Work out the finished part from the listing and answer in its coordinate system (mm). Face numbers are marked on the shaded views. A direction names the side the tool comes from. Give positions to 0.01 mm unless a question says otherwise; leave off trailing zeros. Loops run counter-clockwise (first coordinate to the right, second up) from the corner with the lowest first, then second, coordinate; pieces in that order, holes last. Notation, with made-up numbers: M -21,78.25 L 3,78.25 A14 cw 3,86.25 Z; hole C 53.25,20 d10. An arc over 180 degrees is marked long. Write item = value, one per line. Start each with the question number.
1. For the marked faces 4, 5, 6 and 7, determine the directions among +Z, -Z, +X, -X, +Y, -Y from which every point of the face is accessible in a straight line to the end or side of a thin tool.
2. Section D-D on x = 4.75 is taken. Determine the outline of the cut face in (y, z), plus the area to 3 significant figures.
3. Section A-A on x = 0 is taken. Determine the outline of the cut face in (y, z) (3 decimals), plus the area to 3 significant figures.
4. Flat-ended cylindrical pins translate along their axes: pin 1 Ø1.6 at (x, z) = (-5.5, 8.5) entering from +Y; pin 2 Ø1.5 at (x, y) = (4.5, 1.5) entering from +Z; pin 3 Ø0.8 at (y, z) = (4, -5) entering from -X. Find the tip coordinate at first contact, or state that the pin passes through.
5. Consider L1, parallel to Z at x = 4.75, y = 3.3; L2, parallel to Z at x = 2.25, y = 4.2; L3, parallel to X at y = 1.15, z = 0 (3 decimals). Determine where each line is inside the solid, lowest interval first. Write a range as [from, to].
6. Section C-C on z = 10.5 is taken. Determine the outline of the cut face in (x, y).
7. The mould has two halves that part along Z. Classify the marked faces 1, 2 and 3: released by +Z, released by -Z, zero draft, split by the parting line, or undercut.
8. Section B-B on z = 3.5 is taken. Determine the outline of the cut face in (x, y).
```python
from build123d import *

# Parameters (mm, degrees)
CROQUIS1_W              = 20
CROQUIS1_H              = 20
SALIENTE_EXTRUIR1_DEPTH = 3
CROQUIS2_W              = 14
CROQUIS2_H              = 14
SALIENTE_EXTRUIR2_DEPTH = 2
CROQUIS3_W              = 12
CROQUIS3_H              = 12
CORTAR_EXTRUIR1_DEPTH   = 2
CROQUIS4_W              = 6
CROQUIS4_H              = 2.600399467
CORTAR_EXTRUIR2_DEPTH   = 3
SALIENTE_EXTRUIR3_DEPTH = 3
CROQUIS6_W              = 3
CROQUIS6_H              = 3
CROQUIS6_W_2            = 2
CROQUIS6_H_2            = 2
CROQUIS6_W_3            = 4
SALIENTE_EXTRUIR4_DEPTH = 0.5
CROQUIS7_W              = 6
CROQUIS7_H              = 2.831475003
CORTAR_EXTRUIR3_DEPTH   = 1
CROQUIS8_W              = 1
CROQUIS8_H              = 5.440516932
SALIENTE_EXTRUIR5_DEPTH = 0.5
CROQUIS10_W             = 3
CROQUIS10_H             = 4.43187447
CROQUIS10_W_2           = 2
CROQUIS10_H_2           = 3.43187447
CROQUIS10_H_3           = 3.13625106
CROQUIS10_H_4           = 2.13625106
CROQUIS10_H_5           = 2.43247793
CROQUIS10_H_6           = 1.43247793
CROQUIS10_W_3           = 1.053408661
CROQUIS10_W_4           = 3.858734252
CROQUIS10_W_5           = 5
CROQUIS10_W_6           = 2.087857087
CROQUIS10_W_7           = 1.087857087
CROQUIS10_H_7           = 1.99939654
CROQUIS10_H_8           = 0.99939654
SALIENTE_EXTRUIR6_DEPTH = 1.5
CROQUIS11_W             = 6
CROQUIS11_H             = 5.43187447
SALIENTE_EXTRUIR7_DEPTH = 1.5
CROQUIS12_R             = 1.575
CORTAR_EXTRUIR4_DEPTH   = 2.5


with BuildPart() as part:
    # Croquis1 → Saliente-Extruir1 (new body)
    with BuildSketch(Plane(origin=(0, 0, 0), x_dir=(1, 0, 0), z_dir=(0, 1, 0))):
        Rectangle(CROQUIS1_W, CROQUIS1_H)
    extrude(amount=SALIENTE_EXTRUIR1_DEPTH)

    # Croquis2 → Saliente-Extruir2 (add)
    with BuildSketch(Plane(origin=(0, 3, 0), x_dir=(1, 0, 0), z_dir=(0, 1, 0))):
        Rectangle(CROQUIS2_W, CROQUIS2_H)
    extrude(amount=SALIENTE_EXTRUIR2_DEPTH)

    # Croquis3 → Cortar-Extruir1 (cut)
    with BuildSketch(Plane(origin=(0, 5, 0), x_dir=(1, 0, 0), z_dir=(0, 1, 0))):
        Rectangle(CROQUIS3_W, CROQUIS3_H)
    extrude(amount=-CORTAR_EXTRUIR1_DEPTH, mode=Mode.SUBTRACT)

    # Croquis4 → Cortar-Extruir2 (cut)
    with BuildSketch(Plane(origin=(0, 5, 0), x_dir=(1, 0, 0), z_dir=(0, 1, 0))):
        with Locations((0, -5.699800267)):
            Rectangle(CROQUIS4_W, CROQUIS4_H)
    extrude(amount=-CORTAR_EXTRUIR2_DEPTH, mode=Mode.SUBTRACT)

    # Croquis5 → Saliente-Extruir3 (add)
    with BuildSketch(Plane(origin=(0, 0, 0), x_dir=(1, 0, 0), z_dir=(0, 1, 0))):
        Polygon((-3, -10), (-1.049339158, -10), (-1.049339158, -14.469917755), (-2.287906915, -14.469917755), align=None)
        Polygon((0.678136925, -10), (3, -10), (1.818923018, -14.469917755), (0.678136925, -14.469917755), align=None)
    extrude(amount=SALIENTE_EXTRUIR3_DEPTH)

    # Croquis6 → Saliente-Extruir4 (add)
    # profile 1 of 4: a face of its own
    with BuildSketch(Plane(origin=(0, 3, 0), x_dir=(1, 0, 0), z_dir=(0, 1, 0))):
        with Locations((-8.5, -8.5)):
            Rectangle(CROQUIS6_W, CROQUIS6_H)
        with Locations((-8.5, -8.5)):
            Rectangle(CROQUIS6_W_2, CROQUIS6_H_2, mode=Mode.SUBTRACT)
    # profile 2 of 4: a face of its own
    with BuildSketch(Plane(origin=(0, 3, 0), x_dir=(1, 0, 0), z_dir=(0, 1, 0))):
        with Locations((-5, -8.5)):
            Rectangle(CROQUIS6_W_3, CROQUIS6_H)
        with Locations((-5, -8.5)):
            Rectangle(CROQUIS6_W, CROQUIS6_H_2, mode=Mode.SUBTRACT)
    # profile 3 of 4: a face of its own
    with BuildSketch(Plane(origin=(0, 3, 0), x_dir=(1, 0, 0), z_dir=(0, 1, 0))):
        with Locations((5, -8.5)):
            Rectangle(CROQUIS6_W_3, CROQUIS6_H)
        with Locations((5, -8.5)):
            Rectangle(CROQUIS6_W, CROQUIS6_H_2, mode=Mode.SUBTRACT)
    # profile 4 of 4: a face of its own
    with BuildSketch(Plane(origin=(0, 3, 0), x_dir=(1, 0, 0), z_dir=(0, 1, 0))):
        with Locations((8.5, -8.5)):
            Rectangle(CROQUIS6_W, CROQUIS6_H)
        with Locations((8.5, -8.5)):
            Rectangle(CROQUIS6_W_2, CROQUIS6_H_2, mode=Mode.SUBTRACT)
    extrude(amount=SALIENTE_EXTRUIR4_DEPTH)

    # Croquis7 → Cortar-Extruir3 (cut)
    with BuildSketch(Plane(origin=(0, 3, 0), x_dir=(1, 0, 0), z_dir=(0, 1, 0))):
        with Locations((0, -2.983863032)):
            Rectangle(CROQUIS7_W, CROQUIS7_H)
    extrude(amount=-CORTAR_EXTRUIR3_DEPTH, mode=Mode.SUBTRACT)

    # Croquis8 → Saliente-Extruir5 (add)
    with BuildSketch(Plane(origin=(0, 3, 0), x_dir=(1, 0, 0), z_dir=(0, 1, 0))):
        with Locations((-2.5, -4.288383996)):
            Rectangle(CROQUIS8_W, CROQUIS8_H)
    extrude(amount=-SALIENTE_EXTRUIR5_DEPTH)

    # Croquis10 → Saliente-Extruir6 (add)
    # profile 1 of 10: a face of its own
    with BuildSketch(Plane(origin=(0, 3, 0), x_dir=(1, 0, 0), z_dir=(0, 1, 0))):
        with Locations((-4.5, -3.784062765)):
            Rectangle(CROQUIS10_W, CROQUIS10_H)
        with Locations((-4.5, -3.784062765)):
            Rectangle(CROQUIS10_W_2, CROQUIS10_H_2, mode=Mode.SUBTRACT)
    # profile 2 of 10: a face of its own
    with BuildSketch(Plane(origin=(0, 3, 0), x_dir=(1, 0, 0), z_dir=(0, 1, 0))):
        with Locations((-4.5, 0)):
            Rectangle(CROQUIS10_W, CROQUIS10_H_3)
        with Locations((-4.5, 0)):
            Rectangle(CROQUIS10_W_2, CROQUIS10_H_4, mode=Mode.SUBTRACT)
    # profile 3 of 10: a face of its own
    with BuildSketch(Plane(origin=(0, 3, 0), x_dir=(1, 0, 0), z_dir=(0, 1, 0))):
        with Locations((-4.5, 2.784364495)):
            Rectangle(CROQUIS10_W, CROQUIS10_H_5)
        with Locations((-4.5, 2.784364495)):
            Rectangle(CROQUIS10_W_2, CROQUIS10_H_6, mode=Mode.SUBTRACT)
    # profile 4 of 10: a face of its own
    with BuildSketch(Plane(origin=(0, 3, 0), x_dir=(1, 0, 0), z_dir=(0, 1, 0))):
        Polygon((-0.946591339, 6), (-3, 6), (-3, 4.00060346), (-3, 1.56812553), (-0.946591339, 1.56812553), align=None)
        with Locations((-1.97329567, 3.784062765)):
            Rectangle(CROQUIS10_W_3, CROQUIS10_H_2, mode=Mode.SUBTRACT)
    # profile 5 of 10: a face of its own
    with BuildSketch(Plane(origin=(0, 3, 0), x_dir=(1, 0, 0), z_dir=(0, 1, 0))):
        Polygon((3.912142913, 6), (-0.946591339, 6), (-0.946591339, 1.56812553), (3, 1.56812553), (3.912142913, 1.56812553), align=None)
        with Locations((1.482775787, 3.784062765)):
            Rectangle(CROQUIS10_W_4, CROQUIS10_H_2, mode=Mode.SUBTRACT)
    # profile 6 of 10: a face of its own
    with BuildSketch(Plane(origin=(0, 3, 0), x_dir=(1, 0, 0), z_dir=(0, 1, 0))):
        Polygon((-0.946591339, 1.56812553), (-3, 1.56812553), (-3, -1.56812553), (3, -1.56812553), (3, 1.56812553), align=None)
        Rectangle(CROQUIS10_W_5, CROQUIS10_H_4, mode=Mode.SUBTRACT)
    # profile 7 of 10: a face of its own
    with BuildSketch(Plane(origin=(0, 3, 0), x_dir=(1, 0, 0), z_dir=(0, 1, 0))):
        with Locations((4.956071457, 3.784062765)):
            Rectangle(CROQUIS10_W_6, CROQUIS10_H)
        with Locations((4.956071457, 3.784062765)):
            Rectangle(CROQUIS10_W_7, CROQUIS10_H_2, mode=Mode.SUBTRACT)
    # profile 8 of 10: a face of its own
    with BuildSketch(Plane(origin=(0, 3, 0), x_dir=(1, 0, 0), z_dir=(0, 1, 0))):
        Polygon((3.912142913, 1.56812553), (3, 1.56812553), (3, -1.56812553), (6, -1.56812553), (6, 1.56812553), align=None)
        with Locations((4.5, 0)):
            Rectangle(CROQUIS10_W_2, CROQUIS10_H_4, mode=Mode.SUBTRACT)
    # profile 9 of 10: a face of its own
    with BuildSketch(Plane(origin=(0, 3, 0), x_dir=(1, 0, 0), z_dir=(0, 1, 0))):
        with Locations((4.5, -3.784062765)):
            Rectangle(CROQUIS10_W, CROQUIS10_H)
        with Locations((4.5, -3.784062765)):
            Rectangle(CROQUIS10_W_2, CROQUIS10_H_2, mode=Mode.SUBTRACT)
    # profile 10 of 10: a face of its own
    with BuildSketch(Plane(origin=(0, 3, 0), x_dir=(1, 0, 0), z_dir=(0, 1, 0))):
        with Locations((-4.5, 5.00030173)):
            Rectangle(CROQUIS10_W, CROQUIS10_H_7)
        with Locations((-4.5, 5.00030173)):
            Rectangle(CROQUIS10_W_2, CROQUIS10_H_8, mode=Mode.SUBTRACT)
    extrude(amount=SALIENTE_EXTRUIR6_DEPTH)

    # Croquis11 → Saliente-Extruir7 (add)
    with BuildSketch(Plane(origin=(0, 2, 0), x_dir=(1, 0, 0), z_dir=(0, 1, 0))):
        with Locations((0, -4.284062765)):
            Rectangle(CROQUIS11_W, CROQUIS11_H)
    extrude(amount=SALIENTE_EXTRUIR7_DEPTH)

    # Croquis12 → Cortar-Extruir4 (cut)
    with BuildSketch(Plane.XZ):
        with Locations(Location((0, 0, 0), (0, 0, 270))):
            Circle(CROQUIS12_R)
    extrude(amount=-CORTAR_EXTRUIR4_DEPTH, mode=Mode.SUBTRACT)


solid = part.part
```
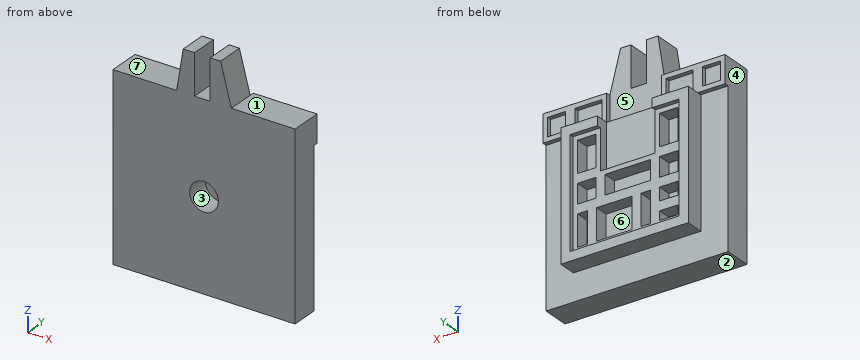
Verdict:
q1.face_4 = +Z, -Z, -X, +Y, -Y
q1.face_5 = +Z, +Y
q1.face_6 = +Y
q1.face_7 = +Z, -X, +Y, -Y
q2.outline = M 0,-10 L 3,-10 L 3,-7 L 5,-7 L 5,-6 L 4.5,-6 L 4.5,-5.5 L 3,-5.5 L 3,-2.07 L 4.5,-2.07 L 4.5,-1.07 L 3,-1.07 L 3,1.07 L 4.5,1.07 L 4.5,2.07 L 3,2.07 L 3,5.5 L 4.5,5.5 L 4.5,6 L 5,6 L 5,7 L 3.5,7 L 3.5,7.5 L 3,7.5 L 3,9.5 L 3.5,9.5 L 3.5,10 L 0,10 Z
q2.area = 69.0 mm2
q3.outline = M 0,-10 L 3,-10 L 3,-7 L 5,-7 L 5,-6 L 4.5,-6 L 4.5,-5.5 L 3,-5.5 L 3,-2.068 L 4.5,-2.068 L 4.5,-1.068 L 3,-1.068 L 3,1.068 L 4.5,1.068 L 4.5,1.568 L 3.5,1.568 L 3.5,7 L 3,7 L 3,10 L 0,10 L 0,1.575 L 2.5,1.575 L 2.5,-1.575 L 0,-1.575 Z
q3.area = 59.8 mm2
q4.pin_1 = 3
q4.pin_2 = 10
q4.pin_3 = -7
q5.L1 = [-7, -5.5], [-2.07, -1.07], [1.07, 2.07], [5.5, 7.5], [9.5, 10]
q5.L2 = [-7, -5.5], [-2.07, -1.07], [1.07, 1.57]
q5.L3 = [-10, -1.575], [1.575, 10]
q6.outline = M -2.92,0 L -1.05,0 L -1.05,3 L -2.92,3 Z; M 0.68,0 L 2.87,0 L 2.87,3 L 0.68,3 Z
q7.face_1 = released by +Z
q7.face_2 = released by -Z
q7.face_3 = undercut
q8.outline = M -10,0 L 10,0 L 10,3 L 7,3 L 7,5 L 6,5 L 6,4.5 L 5.5,4.5 L 5.5,3 L 3.5,3 L 3.5,4.5 L 3,4.5 L 3,3.5 L -3,3.5 L -3,4.5 L -3.5,4.5 L -3.5,3 L -5.5,3 L -5.5,4.5 L -6,4.5 L -6,5 L -7,5 L -7,3 L -10,3 Z
